```python
from build123d import *

# Parameters (mm, degrees)
F0_R     = 2.54
F1_DEPTH = 3.175


with BuildPart() as f1:
    # F0 (on Top) → F1 (new body)
    with BuildSketch(Plane.XY):
        with BuildLine():
            ThreePointArc((0, 12.7), (-8.980256, -8.980256), (12.7, 0))
            Line((12.7, 0), (444.5, 0))
            ThreePointArc((444.5, 0), (466.180256, -8.980256), (457.2, 12.7))
            Line((457.2, 12.7), (457.2, 114.3))
            ThreePointArc((457.2, 114.3), (466.180256, 135.980256), (444.5, 127))
            Line((444.5, 127), (12.7, 127))
            ThreePointArc((12.7, 127), (-8.980256, 135.980256), (0, 114.3))
            Line((0, 114.3), (0, 12.7))
        make_face()
        Circle(F0_R, mode=Mode.SUBTRACT)
        with BuildLine():
            Line((57.15, 95.25), (57.15, 31.75))
            ThreePointArc((57.15, 31.75), (50.8, 25.4), (44.45, 31.75))
            Line((44.45, 31.75), (44.45, 95.25))
            ThreePointArc((44.45, 95.25), (50.8, 101.6), (57.15, 95.25))
        make_face(mode=Mode.SUBTRACT)
        with BuildLine():
            Line((88.9, 31.75), (88.9, 95.25))
            ThreePointArc((88.9, 95.25), (95.25, 101.6), (101.6, 95.25))
            Line((101.6, 95.25), (101.6, 31.75))
            ThreePointArc((101.6, 31.75), (95.25, 25.4), (88.9, 31.75))
        make_face(mode=Mode.SUBTRACT)
        with BuildLine():
            Line((133.35, 31.75), (133.35, 95.25))
            ThreePointArc((133.35, 95.25), (139.7, 101.6), (146.05, 95.25))
            Line((146.05, 95.25), (146.05, 31.75))
            ThreePointArc((146.05, 31.75), (139.7, 25.4), (133.35, 31.75))
        make_face(mode=Mode.SUBTRACT)
        with BuildLine():
            Line((177.8, 31.75), (177.8, 95.25))
            ThreePointArc((177.8, 95.25), (184.15, 101.6), (190.5, 95.25))
            Line((190.5, 95.25), (190.5, 31.75))
            ThreePointArc((190.5, 31.75), (184.15, 25.4), (177.8, 31.75))
        make_face(mode=Mode.SUBTRACT)
        with Locations((457.2, 0)):
            Circle(F0_R, mode=Mode.SUBTRACT)
        with BuildLine():
            Line((222.25, 31.75), (222.25, 95.25))
            ThreePointArc((222.25, 95.25), (228.6, 101.6), (234.95, 95.25))
            Line((234.95, 95.25), (234.95, 31.75))
            ThreePointArc((234.95, 31.75), (228.6, 25.4), (222.25, 31.75))
        make_face(mode=Mode.SUBTRACT)
        with BuildLine():
            Line((266.7, 31.75), (266.7, 95.25))
            ThreePointArc((266.7, 95.25), (273.05, 101.6), (279.4, 95.25))
            Line((279.4, 95.25), (279.4, 31.75))
            ThreePointArc((279.4, 31.75), (273.05, 25.4), (266.7, 31.75))
        make_face(mode=Mode.SUBTRACT)
        with BuildLine():
            Line((311.15, 31.75), (311.15, 95.25))
            ThreePointArc((311.15, 95.25), (317.5, 101.6), (323.85, 95.25))
            Line((323.85, 95.25), (323.85, 31.75))
            ThreePointArc((323.85, 31.75), (317.5, 25.4), (311.15, 31.75))
        make_face(mode=Mode.SUBTRACT)
        with BuildLine():
            Line((355.6, 31.75), (355.6, 95.25))
            ThreePointArc((355.6, 95.25), (361.95, 101.6), (368.3, 95.25))
            Line((368.3, 95.25), (368.3, 31.75))
            ThreePointArc((368.3, 31.75), (361.95, 25.4), (355.6, 31.75))
        make_face(mode=Mode.SUBTRACT)
        with BuildLine():
            Line((400.05, 31.75), (400.05, 95.25))
            ThreePointArc((400.05, 95.25), (406.4, 101.6), (412.75, 95.25))
            Line((412.75, 95.25), (412.75, 31.75))
            ThreePointArc((412.75, 31.75), (406.4, 25.4), (400.05, 31.75))
        make_face(mode=Mode.SUBTRACT)
        with Locations((0, 127)):
            Circle(F0_R, mode=Mode.SUBTRACT)
        with Locations((457.2, 127)):
            Circle(F0_R, mode=Mode.SUBTRACT)
    extrude(amount=F1_DEPTH)


solid = f1.part
```
CAD build for the part. Positions are in the model's coordinates, mm. Coordinates: 2 decimals unless noted, no trailing zeros. Order: outer loops, then holes, each group sorted by start corner. A loop starts at its lowest first (then second) coordinate and runs counter-clockwise, first axis right, second up. Notation, with made-up numbers: (-2.5, 20) -> (20.5, 20) arc R21 cw to (20.5, 47) -> close; hole circle Ø11 at (76.25, 57.25). An arc over 180 degrees is marked (long way). Use one line per item in the form item = value. Start each with the question number.
1) Pull direction Y, two halves, no side cores. Call faces 1 (the cylindrical face through (466.47, 135.68, 1.57)), 2 (the flat face through (172, 65, 3.175)): +Y half, -Y half, draft (parallel to the pull), parting line (faces both ways), or undercut.
2) Band-saw the part on B-B on y = 79.5. State how many separate pieces and enclosed holes the cut face has, then the cut area to 3 significant figures.
3) Drill centre lines: L1, parallel to Y at x = 374.5, z = 1.8; L2, parallel to X at y = -1, z = 2.8; L3, parallel to X at y = 103.5, z = 0.55. Where is each one in solid material? Low to high. Write a range as [from, to].
4) Band-saw the part on A-A on x = 50.8. Give the cut face in (y, z) (3 decimals).
5) Band-saw the part on D-D on x = 427. Give the cut face in (y, z) (3 decimals).
6) Drop flat-ended pins along their axis: pin 1 (1 mm diameter, centred on y = 65.5, z = 2.5, fed in from +X); pin 2 (1 mm diameter, centred on x = 198, z = 1, fed in from +Y); pin 3 (1 mm diameter, centred on y = 65, z = 2, fed in from -X). Give the stop position or say it passes through.
Entries:
q1.face_1 = undercut
q1.face_2 = draft
q2.separate_pieces = 10
q2.enclosed_holes = 0
q2.area = 1,090 mm2
q3.L1 = [0, 127]
q3.L2 = [-12.66, -2.33], [2.33, 12.66], [444.54, 454.87], [459.53, 469.86]
q3.L3 = [0, 457.2]
q4.outline = (0, 0) -> (25.4, 0) -> (25.4, 3.175) -> (0, 3.175) -> close; (101.6, 0) -> (127, 0) -> (127, 3.175) -> (101.6, 3.175) -> close
q5.outline = (0, 0) -> (127, 0) -> (127, 3.175) -> (0, 3.175) -> close
q6.pin_1 = 457.2
q6.pin_2 = 127
q6.pin_3 = 0
